The model under review builds one solid part; all positions refer to its coordinate system, in mm. Round coordinates to 2 decimals unless told otherwise and drop trailing zeros. Write each loop counter-clockwise with the first axis right and the second up, starting at its lowest first coordinate (ties: lowest second). Pieces come first, ordered by that corner, then holes. Notation, with made-up numbers: (-27, 19.5) - (-20, 19.5) arc R17 ccw to (-20, 51.5) - close; hole circle Ø2 at (-33.75, 83). An arc over 180 degrees is marked (long way). Return JSON: item names as keys, results as strings.
from build123d import *

# Parameters (mm, degrees)
F0_R     = 12.7
F0_R_2   = 11.2
F1_DEPTH = 457.2
F2_R     = 3.175
F3_DEPTH = 12.7


with BuildPart() as f1:
    # F0 (on Top) → F1 (new body)
    with BuildSketch(Plane.XY):
        Circle(F0_R)
        Circle(F0_R_2, mode=Mode.SUBTRACT)
    extrude(amount=F1_DEPTH)

    # F2 (on Front) → F3 (cut, symmetric)
    with BuildSketch(Plane.XZ):
        with Locations((0, 76.2)):
            Circle(F2_R)
        with Locations((0, 228.6)):
            Circle(F2_R)
        with Locations((0, 101.6)):
            Circle(F2_R)
    extrude(amount=F3_DEPTH, both=True, mode=Mode.SUBTRACT)


solid = f1.part
(1) Add section B-B (z = 144.5). Write out the cut boundary in (x, y), plus the area to 3 significant figures.
Filled in:
{"outline": "circle Ø25.4 at (0, 0); hole circle Ø22.4 at (0, 0)", "area": "113 mm2"}
(2) Add section A-A (x = 7). Write out the cut boundary in (y, z), plus the area to 3 significant figures.
Filled in:
{"outline": "(-10.6, 0) - (-8.74, 0) - (-8.74, 457.2) - (-10.6, 457.2) - close; (8.74, 0) - (10.6, 0) - (10.6, 457.2) - (8.74, 457.2) - close", "area": "1,700 mm2"}
(3) Add section C-C (y = -4.75). Write out the cut boundary in (x, z).
Filled in:
{"outline": "(-11.78, 0) - (-10.14, 0) - (-10.14, 457.2) - (-11.78, 457.2) - close; (10.14, 0) - (11.78, 0) - (11.78, 457.2) - (10.14, 457.2) - close"}
(4) Mouldability with a two-part tool opening along X and no side actions: class faces 1 (the flat face through (7, -9, 0)), 2 (the cylindrical face through (-2.75, -12.4, 225.4)), 3 (the cylindrical face through (-11.19, 0.49, 225.4)) as released by +X, released by -X, zero draft, split by the parting line, or undercut.
Filled in:
{"face 1": "zero draft", "face 2": "split by the parting line", "face 3": "undercut"}
(5) Wall thickness on line 1 (Z direction, x = 0, y = -11.75) (3 decimals); line 2 (X direction, y = -1, z = 240); line 3 (Y direction, x = -0.5, z = 90.5): over which ranges is each line inside the solid? List them lowest first.
Filled in:
{"line 1": "z = 0 to 73.025, 79.375 to 98.425, 104.775 to 225.425, 231.775 to 457.2", "line 2": "x = -12.66 to -11.16, 11.16 to 12.66", "line 3": "y = -12.69 to -11.19, 11.19 to 12.69"}
(6) Clearance check with flat-ended pins moving along their axes: pin 1 Ø5 at (x, z) = (4, 221.5) entering from -Y; pin 2 Ø8 at (x, z) = (-7, 391.5) entering from -Y; pin 3 Ø6 at (y, z) = (9.5, 256) entering from +X. State where each tip first meets the part, or that it passes through.
Filled in:
{"pin 1": "stops at y = -12.61", "pin 2": "stops at y = -12.34", "pin 3": "stops at x = 10.91"}
